```python
from build123d import *

# Parameters (mm, degrees)
SALIENTE_EXTRUIR1_DEPTH = 3
CROQUIS2_R              = 2.38125
CORTAR_EXTRUIR1_DEPTH   = 4


with BuildPart() as part:
    # Croquis1 → Saliente-Extruir1 (new body)
    with BuildSketch(Plane.XY):
        Polygon((75, 0), (-75, 0), (0, 150), align=None)
    extrude(amount=SALIENTE_EXTRUIR1_DEPTH)

    # Croquis2 → Cortar-Extruir1 (cut, through all)
    with BuildSketch(Plane.XY):
        with Locations((0, 128)):
            Circle(CROQUIS2_R)
        Polygon((5, 140), (0, 150), (-5, 140), align=None)
    extrude(amount=CORTAR_EXTRUIR1_DEPTH, mode=Mode.SUBTRACT)


solid = part.part
```
Check sheet for the modelled part. Datum: model origin and axes. Units: mm. Round coordinates to 2 decimals unless told otherwise and drop trailing zeros. Order: outer loops, then holes, each group sorted by start corner. A loop starts at its lowest first (then second) coordinate and runs counter-clockwise, first axis right, second up. Notation, with made-up numbers: (80, -30.5) - (107, -30.5) arc R20 ccw to (107, -23.5) - close; hole circle Ø9 at (11, 63.25). An arc over 180 degrees is marked (long way). Write item = value, one per line.
Q1. Draft check along Y on faces 1 (the face through (-0.31, 130.36, 1.48)), 2 (the face through (-40.5, 69, 1.5)), 3 (the face through (1, 55, 0)). Enter one of: pulls with the +Y half, pulls with the -Y half, needs draft (parallel to the pull), parting line crosses it, or undercut.
Computed:
face_1 = undercut
face_2 = pulls with the +Y half
face_3 = needs draft
Q2. Section check D-D (x = 54). Record the boundary of the cut face in (y, z), and give its area (3 significant figures).
Computed:
outline = (0, 0) - (42, 0) - (42, 3) - (0, 3) - close
area = 126 mm^2
Q3. Go/stop test with flat-tipped pins: pin 1 (5 mm diameter, centred on x = -5, y = 60, fed in from -Z); pin 2 (1 mm diameter, centred on x = 26, z = 1, fed in from +Y); pin 3 (4.5 mm diameter, centred on x = 0, y = 128, fed in from +Z). Record where each tip stops, or that it passes through.
Computed:
pin_1 = 0
pin_2 = 99
pin_3 = through
Q4. Thickness scan on line 1 along Y through (x, z) = (0, 1.25); line 2 along X through (y, z) = (128, 1.4); line 3 along X through (y, z) = (128.5, 1.9). Record the ranges inside material, lowest first.
Computed:
line_1 = 0 to 125.62, 130.38 to 140
line_2 = -11 to -2.38, 2.38 to 11
line_3 = -10.75 to -2.33, 2.33 to 10.75
Q5. Section check A-A (y = 128). Record the boundary of the cut face in (x, z), and give its area (3 significant figures).
Computed:
outline = (-11, 0) - (-2.38, 0) - (-2.38, 3) - (-11, 3) - close; (2.38, 0) - (11, 0) - (11, 3) - (2.38, 3) - close
area = 51.7 mm^2
Q6. Section check C-C (z = 1). Record the boundary of the cut face in (x, y), and give its area (3 significant figures).
Computed:
outline = (-75, 0) - (75, 0) - (5, 140) - (-5, 140) - close; hole circle Ø4.76 at (0, 128)
area = 11,200 mm^2
Q7. Section check B-B (x = 0). Record the boundary of the cut face in (y, z), and give its area (3 significant figures).
Computed:
outline = (0, 0) - (125.62, 0) - (125.62, 3) - (0, 3) - close; (130.38, 0) - (140, 0) - (140, 3) - (130.38, 3) - close
area = 406 mm^2
